```python
from build123d import *

# Parameters (mm, degrees)
EXTRUDE_THIN1_DEPTH        = 38.1
F_10_0MM_DOWEL_HOLE1_D     = 12.7
F_10_0MM_DOWEL_HOLE1_DEPTH = 6.35
F_10_0MM_DOWEL_HOLE1_TIP   = 3.815464931
F_10_0MM_DOWEL_HOLE2_D     = 9.53
F_10_0MM_DOWEL_HOLE2_DEPTH = 6.35
F_10_0MM_DOWEL_HOLE2_TIP   = 2.86310085


with BuildPart() as part:
    # Sketch1 → Extrude-Thin1 (new body)
    with BuildSketch(Plane.XY):
        with BuildLine():
            Line((-63.51, 47.625), (-9.52, 47.625))
            ThreePointArc((-9.52, 47.625), (-2.788343443, 44.836656557), (0, 38.105))
            Line((0, 38.105), (0, -38.105))
            ThreePointArc((0, -38.105), (-2.788343443, -44.836656557), (-9.52, -47.625))
            Line((-9.52, -47.625), (-50.651363667, -47.625))
            ThreePointArc((-50.651363667, -47.625), (-53.910815633, -47.050270676), (-56.777129588, -45.395403543))
            Line((-56.777129588, -45.395403543), (-88.66094394, -18.641706679))
            Line((-88.66094394, -18.641706679), (-84.579242619, -13.777324465))
            Line((-84.579242619, -13.777324465), (-52.695428266, -40.531021329))
            ThreePointArc((-52.695428266, -40.531021329), (-51.738987723, -41.083222534), (-50.651363667, -41.275))
            Line((-50.651363667, -41.275), (-9.52, -41.275))
            ThreePointArc((-9.52, -41.275), (-7.278471504, -40.346528496), (-6.35, -38.105))
            Line((-6.35, -38.105), (-6.35, 38.105))
            ThreePointArc((-6.35, 38.105), (-7.278471504, 40.346528496), (-9.52, 41.275))
            Line((-9.52, 41.275), (-63.51, 41.275))
            Line((-63.51, 41.275), (-63.51, 47.625))
        make_face()
    extrude(amount=EXTRUDE_THIN1_DEPTH)

    # Ø10.0mm Dowel Hole1
    with Locations(Plane(origin=(0, 47.625, 0), x_dir=(1, 0, 0), z_dir=(0, 1, 0))):
        with Locations((-44.47, -19.05)):
            Hole(F_10_0MM_DOWEL_HOLE1_D / 2, depth=F_10_0MM_DOWEL_HOLE1_DEPTH)
            with Locations((0, 0, -(F_10_0MM_DOWEL_HOLE1_DEPTH + F_10_0MM_DOWEL_HOLE1_TIP / 2))):  # 118° drill point
                Cone(0, F_10_0MM_DOWEL_HOLE1_D / 2, F_10_0MM_DOWEL_HOLE1_TIP, mode=Mode.SUBTRACT)

    # Ø10.0mm Dowel Hole2
    with Locations(Plane(origin=(-45.811814931, -54.596395027, 0), x_dir=(-0.766044443, 0.64278761, 0), z_dir=(-0.64278761, -0.766044443, 0))):
        with Locations((35.12556535, -19.05)):
            Hole(F_10_0MM_DOWEL_HOLE2_D / 2, depth=F_10_0MM_DOWEL_HOLE2_DEPTH)
            with Locations((0, 0, -(F_10_0MM_DOWEL_HOLE2_DEPTH + F_10_0MM_DOWEL_HOLE2_TIP / 2))):  # 118° drill point
                Cone(0, F_10_0MM_DOWEL_HOLE2_D / 2, F_10_0MM_DOWEL_HOLE2_TIP, mode=Mode.SUBTRACT)


solid = part.part
```
Design review of the part built by this model. Coordinates are the model's own, in mm. A direction names the side the tool comes from. Give positions to 0.01 mm unless a question says otherwise; leave off trailing zeros. Write each loop counter-clockwise with the first axis right and the second up, starting at its lowest first coordinate (ties: lowest second). Pieces come first, ordered by that corner, then holes. Notation, with made-up numbers: (5.5, -23) - (31.5, -23) arc R15 ccw to (31.5, 0) - close; hole circle Ø8 at (36, 49). An arc over 180 degrees is marked (long way). Return JSON: item names as keys, results as strings. Group by question number.
(1) Mouldability with a two-part tool opening along Y and no side actions: class faces 6 (the flat face through (-5, 0, 38.1)), 7 (the cylindrical face through (-7.25, 40.32, 18.78)), 8 (the cylindrical face through (-2.71, -44.76, 18.78)) as +Y half, -Y half, draft (parallel to the pull), parting line (faces both ways), or undercut.
(2) To check wall thickness, follow probe 1 along Z at (x, y) = (-44, 45); probe 2 along Y at (x, z) = (-48.5, 11.5) (3 decimals); probe 3 along X at (y, z) = (-18.5, 15). State the ranges of each line that lie inside material, in increasing order.
(3) Insertion check: pin 1 (11.5 mm diameter, centred on x = -44.47, z = 19.05, fed in from +Y) (3 decimals); pin 2 (1 mm diameter, centred on y = -28, z = 16.5, fed in from -X); pin 3 (12 mm diameter, centred on y = 13, z = 6.5, fed in from -X). Each pin has a flat end and moves straight along its axis. Give the tip position at first contact, or say it passes through.
(4) Machinability: for faces 1 (the flat face through (-36, 41.275, 19)), 2 (the flat face through (-86.649, -16.244, 18.783)), 3 (the cylindrical face through (-53.867, -47.066, 18.783)), 4 (the cylindrical face through (-7.3, -40.37, 18.78)), 5 (the cylindrical face through (-50.336, 44.406, 21.482)), which of the approach directions +Z, -Z, +X, -X, +Y, -Y give a long, thin tool a straight path to every point of the face, cutting with its end or side? Answer none if there is none.
(5) We need section D-D, the plane z = 16.5. Give the number of separate pieces and of enclosed holes in the cut face, then the cut area to 3 significant figures.
(6) We need section B-B, the plane x = -44.47. Give the boundary of the cut face in (y, z) (3 decimals).
(7) We need section C-C, the plane z = 4.5. Give the boundary of the cut face in (x, y) (3 decimals), then the cut area to 3 significant figures.
(8) We need section A-A, the plane x = -20.5. Give the boundary of the cut face in (y, z) (3 decimals), then the cut area to 3 significant figures.
Reported:
{
 "1": {"face 6": "draft", "face 7": "undercut", "face 8": "-Y half"},
 "2": {"probe 1": "z = 0 to 12.72, 25.38 to 38.1", "probe 2": "y = -47.625 to -41.275, 41.275 to 47.625", "probe 3": "x = -88.54 to -78.95, -6.35 to 0"},
 "3": {"pin 1": "stops at y = -41.275", "pin 2": "stops at x = -78.1", "pin 3": "stops at x = -6.35"},
 "4": {"face 1": "+Z, -Z, -X", "face 2": "+Z, -Z, -X, +Y", "face 3": "+Z, -Z, -X, -Y", "face 4": "+Z, -Z", "face 5": "+Y"},
 "5": {"separate pieces": "3", "enclosed holes": "0", "area": "1,380 mm2"},
 "6": {"outline": "(-47.625, 0) - (-41.275, 0) - (-41.275, 38.1) - (-47.625, 38.1) - close; (41.275, 0) - (47.625, 0) - (47.625, 12.7) - (41.275, 12.7) - close; (41.275, 25.4) - (47.625, 25.4) - (47.625, 38.1) - (41.275, 38.1) - close"},
 "7": {"outline": "(-88.661, -18.642) - (-56.777, -45.395) arc R9.53 ccw to (-50.651, -47.625) - (-9.52, -47.625) arc R9.52 ccw to (0, -38.105) - (0, 38.105) arc R9.52 ccw to (-9.52, 47.625) - (-63.51, 47.625) - (-63.51, 41.275) - (-9.52, 41.275) arc R3.17 cw to (-6.35, 38.105) - (-6.35, -38.105) arc R3.17 cw to (-9.52, -41.275) - (-50.651, -41.275) arc R3.18 cw to (-52.695, -40.531) - (-84.579, -13.777) - close", "area": "1,510 mm2"},
 "8": {"outline": "(-47.625, 0) - (-41.275, 0) - (-41.275, 38.1) - (-47.625, 38.1) - close; (41.275, 0) - (47.625, 0) - (47.625, 38.1) - (41.275, 38.1) - close", "area": "484 mm2"}
}
